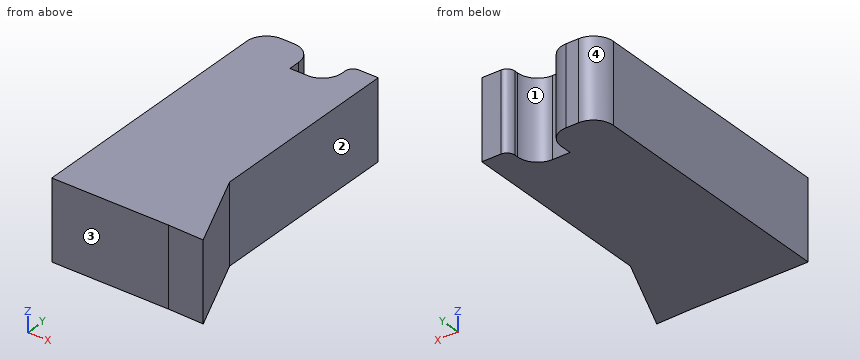
from build123d import *

# Parameters (mm, degrees)
F1_DEPTH = 25.4


with BuildPart() as f1:
    # F0 (on Top) → F1 (new body)
    with BuildSketch(Plane.XY):
        with BuildLine():
            Line((-38.512521, 32.880403), (-42.541664, 32.880403))
            ThreePointArc((-42.541664, 32.880403), (-47.031792, 31.020531), (-48.891664, 26.530403))
            Line((-48.891664, 26.530403), (-48.891664, -56.011409))
            Line((-48.891664, -56.011409), (-11.445787, -56.011409))
            Line((-11.445787, -56.011409), (0, -56.350652))
            Line((0, -56.350652), (-11.445787, -30.049009))
            Line((-11.445787, -30.049009), (-11.445787, 32.880403))
            Line((-11.445787, 32.880403), (-17.630178, 32.880403))
            ThreePointArc((-17.630178, 32.880403), (-19.426229, 32.136454), (-20.170178, 30.340403))
            Line((-20.170178, 30.340403), (-20.170178, 29.141145))
            ThreePointArc((-20.170178, 29.141145), (-22.03005, 24.651017), (-26.520178, 22.791145))
            Line((-26.520178, 22.791145), (-32.162521, 22.791145))
            Line((-32.162521, 22.791145), (-32.162521, 26.530403))
            ThreePointArc((-32.162521, 26.530403), (-34.022393, 31.020531), (-38.512521, 32.880403))
        make_face()
    extrude(amount=F1_DEPTH)


solid = f1.part
Could you check a few things on this model? Use its own coordinates, in mm. Face numbers are marked on the shaded views. A direction names the side the tool comes from. Coordinates: 2 decimals unless noted, no trailing zeros. Order: outer loops, then holes, each group sorted by start corner. A loop starts at its lowest first (then second) coordinate and runs counter-clockwise, first axis right, second up. Notation, with made-up numbers: (1, -30.5) -> (9, -30.5) arc R11 cw to (9, -16.5) -> close; hole circle Ø7 at (36.25, 26). An arc over 180 degrees is marked (long way). One line per item, written item: value. Start each with the question number.
1) I'm going to push flat-ended pins straight in: pin 1 (5 mm diameter, centred on y = 17, z = 22, fed in from +X); pin 2 (12 mm diameter, centred on x = -40, z = 19.5, fed in from -Y); pin 3 (12 mm diameter, centred on y = -42.5, z = 13.5, fed in from +X). Where does each tip first touch, or does it pass through?
2) Imagine slicing it at D-D on x = -3. List the corners of the cut face in (y, z) for me.
3) Which directions (+Z, -Z, +X, -X, +Y, -Y) give clear straight access to the entire face, cutting with the end or side of a thin tool? Please do the marked faces 1, 2, 3 and 4.
4) If I drill on L1, parallel to Y at x = -11.5, z = 21.25; L2, parallel to X at y = -27, z = 13; L3, parallel to X at y = 29.5, z = 6.5, over which ranges is the centre line in solid material (lowest first)? Write a range as [from, to].
5) Imagine slicing it at B-B on z = 4.25. List the corners of the cut face in (x, y) for me.
6) Imagine slicing it at A-A on y = 25.5. List the corners of the cut face in (x, z) for me, plus the area to 3 significant figures.
7) Imagine slicing it at C-C on y = -8. List the corners of the cut face in (x, z) for me.
Answer list:
1. pin 1: stops at x = -11.45
1. pin 2: stops at y = -56.01
1. pin 3: stops at x = -3.42
2. outline: (-56.26, 0) -> (-49.46, 0) -> (-49.46, 25.4) -> (-56.26, 25.4) -> close
3. face 1: +Z, -Z, +Y
3. face 2: +Z, -Z, +X, +Y
3. face 3: +Z, -Z, -X, -Y
3. face 4: +Z, -Z, -X, +Y
4. L1: y = [-56.01, 32.88]
4. L2: x = [-48.89, -11.45]
4. L3: x = [-48.15, -32.9], [-20.17, -11.45]
5. outline: (-48.89, -56.01) -> (-11.45, -56.01) -> (0, -56.35) -> (-11.45, -30.05) -> (-11.45, 32.88) -> (-17.63, 32.88) arc R2.54 ccw to (-20.17, 30.34) -> (-20.17, 29.14) arc R6.35 cw to (-26.52, 22.79) -> (-32.16, 22.79) -> (-32.16, 26.53) arc R6.35 ccw to (-38.51, 32.88) -> (-42.54, 32.88) arc R6.35 ccw to (-48.89, 26.53) -> close
6. outline: (-48.89, 0) -> (-32.16, 0) -> (-32.16, 25.4) -> (-48.89, 25.4) -> close; (-21.32, 0) -> (-11.45, 0) -> (-11.45, 25.4) -> (-21.32, 25.4) -> close
6. area: 676 mm2
7. outline: (-48.89, 0) -> (-11.45, 0) -> (-11.45, 25.4) -> (-48.89, 25.4) -> close
